```python
from build123d import *

# Parameters (mm, degrees)
BOSS_EXTRUDE1_DEPTH = 60
SKETCH1_3_R         = 6.03192879
SKETCH1_3_R_2       = 3.302
BOSS_EXTRUDE2_DEPTH = 30
BOSS_EXTRUDE3_DEPTH = 3.175


with BuildPart() as part:
    # Sketch1 → Boss-Extrude1 (new body)
    with BuildSketch(Plane(origin=(0, 0, 0), x_dir=(1, 0, 0), z_dir=(0, 1, 0))):
        with BuildLine():
            ThreePointArc((17.972934813, -4.85829948), (15.51607121, 0), (17.972934813, 4.85829948))
            Line((17.972934813, 4.85829948), (9.308433067, 4.85829948))
            ThreePointArc((9.308433067, 4.85829948), (7.424621202, 7.424621202), (4.85829948, 9.308433067))
            Line((4.85829948, 9.308433067), (4.85829948, 17.972934813))
            ThreePointArc((4.85829948, 17.972934813), (0, 15.51607121), (-4.85829948, 17.972934813))
            Line((-4.85829948, 17.972934813), (-4.85829948, 9.308433067))
            ThreePointArc((-4.85829948, 9.308433067), (-7.424621202, 7.424621202), (-9.308433067, 4.85829948))
            Line((-9.308433067, 4.85829948), (-17.972934813, 4.85829948))
            ThreePointArc((-17.972934813, 4.85829948), (-15.51607121, 0), (-17.972934813, -4.85829948))
            Line((-17.972934813, -4.85829948), (-9.308433067, -4.85829948))
            ThreePointArc((-9.308433067, -4.85829948), (-7.424621202, -7.424621202), (-4.85829948, -9.308433067))
            Line((-4.85829948, -9.308433067), (-4.85829948, -17.972934813))
            ThreePointArc((-4.85829948, -17.972934813), (0, -15.51607121), (4.85829948, -17.972934813))
            Line((4.85829948, -17.972934813), (4.85829948, -9.308433067))
            ThreePointArc((4.85829948, -9.308433067), (7.424621202, -7.424621202), (9.308433067, -4.85829948))
            Line((9.308433067, -4.85829948), (17.972934813, -4.85829948))
        make_face()
    extrude(amount=BOSS_EXTRUDE1_DEPTH)

    # Sketch1_3 → Boss-Extrude2 (add)
    with BuildSketch(Plane(origin=(0, 0, 0), x_dir=(1, 0, 0), z_dir=(0, 1, 0))):
        with Locations((21.548, 0)):
            Circle(SKETCH1_3_R)
        with Locations((21.548, 0)):
            Circle(SKETCH1_3_R_2, mode=Mode.SUBTRACT)
        with Locations((0, -21.548)):
            Circle(SKETCH1_3_R)
        with Locations((0, -21.548)):
            Circle(SKETCH1_3_R_2, mode=Mode.SUBTRACT)
        with Locations((-21.548, 0)):
            Circle(SKETCH1_3_R)
        with Locations((-21.548, 0)):
            Circle(SKETCH1_3_R_2, mode=Mode.SUBTRACT)
        with Locations((0, 21.548)):
            Circle(SKETCH1_3_R)
        with Locations((0, 21.548)):
            Circle(SKETCH1_3_R_2, mode=Mode.SUBTRACT)
    extrude(amount=BOSS_EXTRUDE2_DEPTH)

    # Sketch2 → Boss-Extrude3 (add)
    with BuildSketch(Plane(origin=(0, 60, 0), x_dir=(1, 0, 0), z_dir=(0, 1, 0))):
        Polygon((5.773502692, 0), (2.886751346, 5), (-2.886751346, 5), (-5.773502692, 0), (-2.886751346, -5), (2.886751346, -5), align=None)
    extrude(amount=BOSS_EXTRUDE3_DEPTH)


solid = part.part
```
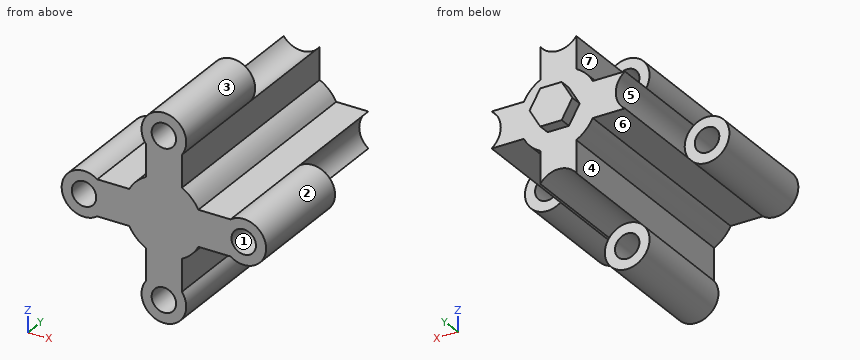
The listing builds one solid part. Answer for the finished solid, in the listing's coordinates (mm). Face numbers are marked on the shaded views. A direction names the side the tool comes from. Coordinates: 2 decimals unless noted, no trailing zeros. Loops run counter-clockwise (first coordinate to the right, second up) from the corner with the lowest first, then second, coordinate; pieces in that order, holes last. Notation, with made-up numbers: (46.25, 83.25) -> (71.25, 83.25) arc R28 ccw to (71.25, 105.25) -> close; hole circle Ø6 at (-9, 74.5). An arc over 180 degrees is marked (long way). Return JSON: item names as keys, results as strings. Group by question number.
(1) A cutting plane is placed at B-B on y = 13. Write down the section's boundary in (x, z), and give its area (3 significant figures).
(2) Find the intervals of material crossed by probe 1 along Z at (x, y) = (0, 12.75); probe 2 along X at (y, z) = (34.5, -12.5), in increasing order. Write a range as from..to.
(3) Given pin 1 Ø4 at (x, z) = (0, -21.548) entering from -Y; pin 2 Ø3 at (x, z) = (5, 6) entering from +Y; pin 3 Ø10.5 at (x, z) = (-21.548, 0) entering from +Y; pin 4 Ø9.5 at (x, y) = (13, 34) entering from -Z, each flat-ended and moving along its own axis, determine where each tip first touches the part or whether it passes through.
(4) Determine the mould class of the marked faces 1, 2, 3 and 4 for opening direction X: released by +X, released by -X, zero draft, split by the parting line, or undercut.
(5) A cutting plane is placed at C-C on z = -19.5. Write down the section's boundary in (x, y), and give its area (3 significant figures).
(6) Which of the six approach directions +Z, -Z, +X, -X, +Y, -Y give full straight-line access (tool end or side, diameter ignored) to the marked faces 5, 6 and 7?
(7) A cutting plane is placed at A-A on x = 0. Write down the section's boundary in (y, z) (3 decimals).
(8) A cutting plane is placed at D-D on y = 34.5. Write down the section's boundary in (x, z).
The answers:
{
 "1": {"outline": "(-17.97, -4.86) -> (-9.31, -4.86) arc R10.5 ccw to (-4.86, -9.31) -> (-4.86, -17.97) arc R6.03 ccw (long way) to (4.86, -17.97) -> (4.86, -9.31) arc R10.5 ccw to (9.31, -4.86) -> (17.97, -4.86) arc R6.03 ccw (long way) to (17.97, 4.86) -> (9.31, 4.86) arc R10.5 ccw to (4.86, 9.31) -> (4.86, 17.97) arc R6.03 ccw (long way) to (-4.86, 17.97) -> (-4.86, 9.31) arc R10.5 ccw to (-9.31, 4.86) -> (-17.97, 4.86) arc R6.03 ccw (long way) to start; hole circle Ø6.6 at (-21.55, 0); hole circle Ø6.6 at (0, -21.55); hole circle Ø6.6 at (0, 21.55); hole circle Ø6.6 at (21.55, 0)", "area": "905 mm^2"},
 "2": {"probe 1": "z = -27.58..-24.85, -18.25..18.25, 24.85..27.58", "probe 2": "x = -4.86..4.86"},
 "3": {"pin 1": "passes through", "pin 2": "stops at y = 60", "pin 3": "stops at y = 30", "pin 4": "stops at z = -6.5"},
 "4": {"face 1": "undercut", "face 2": "undercut", "face 3": "split by the parting line", "face 4": "released by -X"},
 "5": {"outline": "(-5.67, 0) -> (-2.59, 0) -> (-2.59, 30) -> (-5.67, 30) -> close; (2.59, 0) -> (5.67, 0) -> (5.67, 30) -> (2.59, 30) -> close", "area": "185 mm^2"},
 "6": {"face 5": "-X, +Y", "face 6": "-Z, +Y, -Y", "face 7": "-X, +Y, -Y"},
 "7": {"outline": "(0, -27.58) -> (30, -27.58) -> (30, -24.85) -> (0, -24.85) -> close; (0, -18.246) -> (30, -18.246) -> (30, -15.516) -> (60, -15.516) -> (60, -5) -> (63.175, -5) -> (63.175, 5) -> (60, 5) -> (60, 15.516) -> (30, 15.516) -> (30, 18.246) -> (0, 18.246) -> close; (0, 24.85) -> (30, 24.85) -> (30, 27.58) -> (0, 27.58) -> close"},
 "8": {"outline": "(-17.97, -4.86) -> (-9.31, -4.86) arc R10.5 ccw to (-4.86, -9.31) -> (-4.86, -17.97) arc R6.03 cw to (4.86, -17.97) -> (4.86, -9.31) arc R10.5 ccw to (9.31, -4.86) -> (17.97, -4.86) arc R6.03 cw to (17.97, 4.86) -> (9.31, 4.86) arc R10.5 ccw to (4.86, 9.31) -> (4.86, 17.97) arc R6.03 cw to (-4.86, 17.97) -> (-4.86, 9.31) arc R10.5 ccw to (-9.31, 4.86) -> (-17.97, 4.86) arc R6.03 cw to start"}
}
